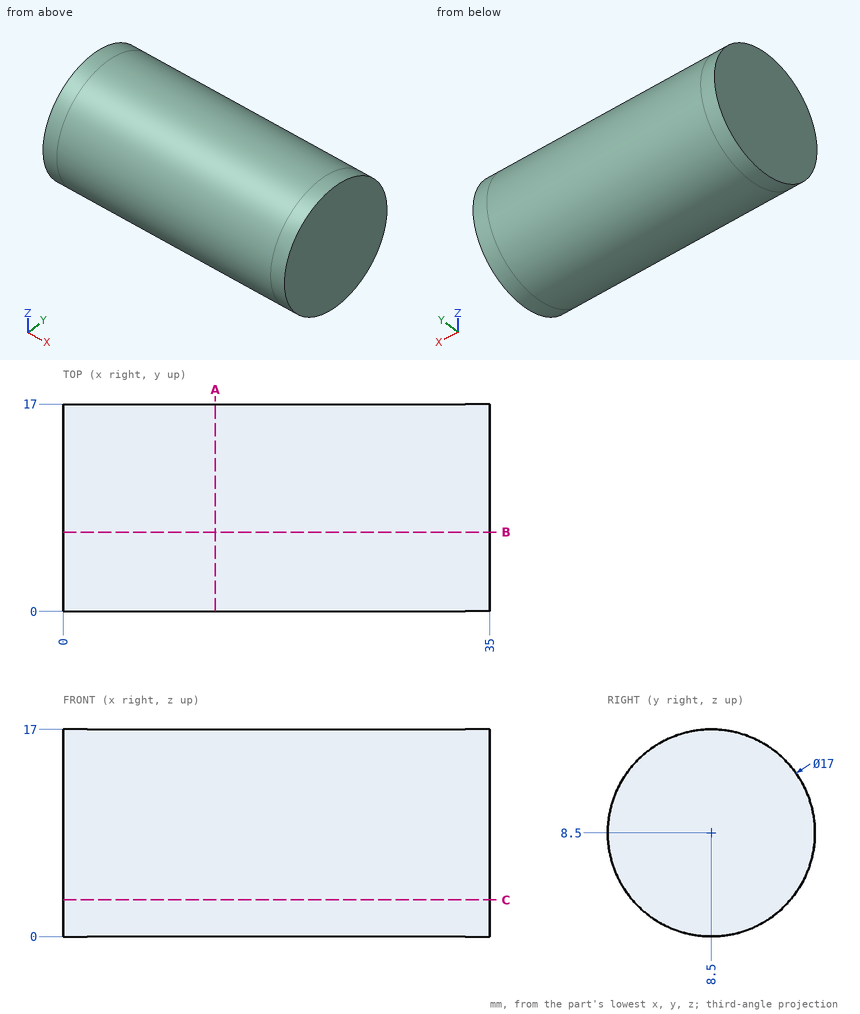
Drawing for the job (mm, zero at the part's lowest x, y, z). Round coordinates to 2 decimals unless told otherwise and drop trailing zeros. Write each loop counter-clockwise with the first axis right and the second up, starting at its lowest first coordinate (ties: lowest second). Pieces come first, ordered by that corner, then holes. Notation, with made-up numbers: (-1, 77) - (13, 77) arc R19 cw to (13, 109) - close; hole circle Ø9 at (22.25, -32). An arc over 180 degrees is marked (long way). Return JSON: item names as keys, results as strings. Group by question number.
Item 1: Flat gauge pins, fed straight in: pin 1 Ø5 at (x, y) = (26, 14) entering from -Z; pin 2 Ø8 at (x, y) = (7, 13) entering from -Z; pin 3 Ø2 at (x, z) = (27, 12.5) entering from +Y. Where does each tip first touch, or does it go through?
Item 2: Band-saw the part on B-B on y = 6.5. List the corners of the cut face in (x, z), plus the area to 3 significant figures.
Item 3: Probe probe 1 along Y at (x, z) = (27.5, 8.25); probe 2 along Z at (x, y) = (31.5, 1); probe 3 along Z at (x, y) = (16, 1.5). List the from-to ranges inside material, lowest first.
Item 4: Band-saw the part on C-C on z = 3. List the corners of the cut face in (x, y).
Item 5: Band-saw the part on A-A on x = 12.5. List the corners of the cut face in (y, z).
Resolved:
{
 "1": {"pin 1": "stops at z = 0.55", "pin 2": "stops at z = 0.01", "pin 3": "stops at y = 16.45"},
 "2": {"outline": "(0, 0.24) - (35, 0.24) - (35, 16.76) - (0, 16.76) - close", "area": "578 mm²"},
 "3": {"probe 1": "y = 0 to 17", "probe 2": "z = 4.5 to 12.5", "probe 3": "z = 3.68 to 13.32"},
 "4": {"outline": "(0, 2.02) - (35, 2.02) - (35, 14.98) - (0, 14.98) - close"},
 "5": {"outline": "circle Ø17 at (8.5, 8.5)"}
}
